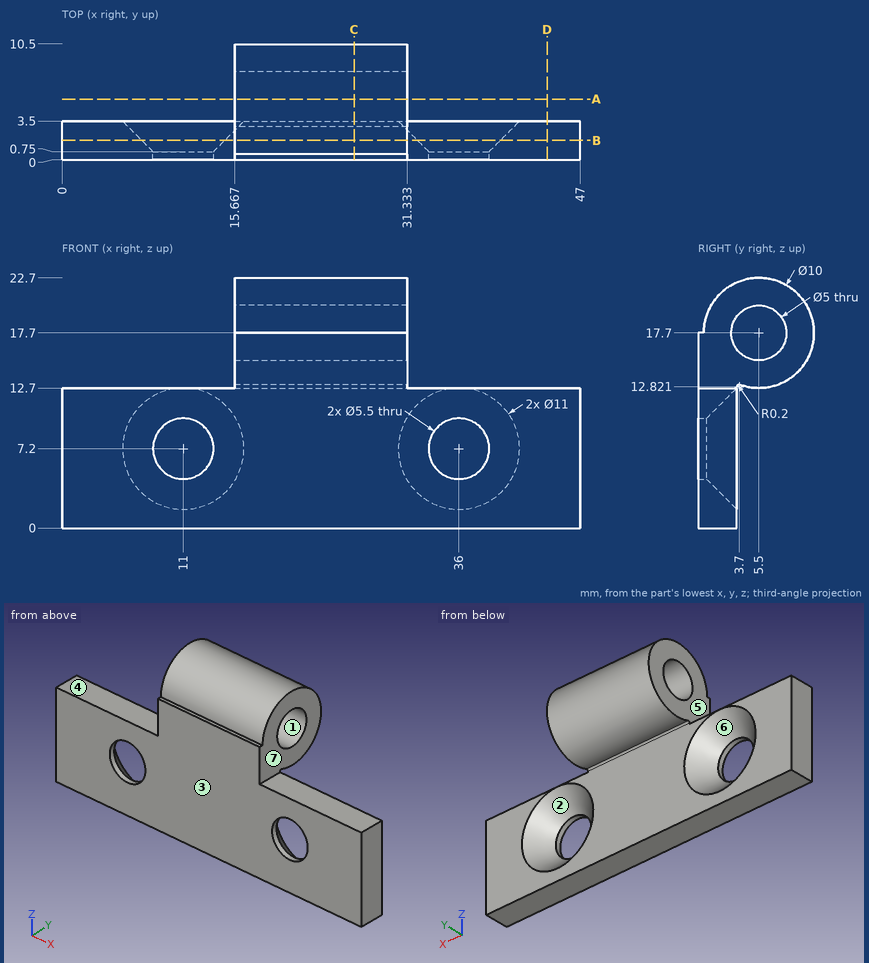
Geometry check sheet. Reference: drawing and pictorial views, mm from the part's lowest x, y, z. A direction names the side the tool comes from. Give positions to 0.01 mm unless a question says otherwise; leave off trailing zeros. Write each loop counter-clockwise with the first axis right and the second up, starting at its lowest first coordinate (ties: lowest second). Pieces come first, ordered by that corner, then holes. Notation, with made-up numbers: (89, 41) - (137, 41) arc R20 cw to (137, 71) - close; hole circle Ø3 at (71.5, 53.5). An arc over 180 degrees is marked (long way). Put each result on its own line as item: value.
Q1. Section check C-C on x = 26.5. Record the cut outline in (y, z), and give its area (3 significant figures).
Result:
outline: (0, 0) - (3.5, 0) - (3.5, 12.82) arc R0.2 cw to (3.77, 13.01) arc R5 ccw (long way) to (0.5, 17.7) - (0, 17.7) - close; hole circle Ø5 at (5.5, 17.7)
area: 111 mm2
Q2. Section check A-A on y = 5.5. Record the cut outline in (x, z).
Result:
outline: (15.67, 12.7) - (31.33, 12.7) - (31.33, 15.2) - (15.67, 15.2) - close; (15.67, 20.2) - (31.33, 20.2) - (31.33, 22.7) - (15.67, 22.7) - close
Q3. Set-up check for the marked faces 5, 6 and 7: record each of +Z, -Z, +X, -X, +Y, -Y from which the full face is reachable in a straight line by a thin tool's end or side.
Result:
face 5: +Z, -X, +Y, -Y
face 6: +Y
face 7: +Z, +X, +Y, -Y
Q4. Depth check by flat-ended pin: P1, Ø6.5, axis at x = 11, z = 7.2, coming from the +Y side; P2, Ø3, axis at x = 12.5, z = 17.5, coming from the -Y side (3 decimals); P3, Ø1.5, axis at y = 9.5, z = 14.5, coming from the -X side; P4, Ø1.8, axis at x = 7.5, y = 1.5, coming from the +Z side. Enter the tip coordinate at first touch or a pass-through.
Result:
P1: y = 1.25
P2: through
P3: x = 15.67
P4: z = 12.7
Q5. Section check B-B on y = 1.75. Record the cut outline in (x, z).
Result:
outline: (0, 0) - (47, 0) - (47, 12.7) - (31.33, 12.7) - (31.33, 21.01) - (15.67, 21.01) - (15.67, 12.7) - (0, 12.7) - close; hole circle Ø7.5 at (11, 7.2); hole circle Ø7.5 at (36, 7.2)
Q6. Scan lines: probe 1 along X at (y, z) = (0.4, 7.2); probe 2 along Z at (x, y) = (11, 0.5); probe 3 along X at (y, z) = (4.25, 21.25). Record each from-to range of solid material in increasing order. Write a range as from..to.
Result:
probe 1: 0..8.25, 13.75..33.25, 38.75..47
probe 2: 0..4.45, 9.95..12.7
probe 3: 15.67..31.33
Q7. Mould release check, pull along Y, two halves, no side actions. Record for the marked faces 1, 2, 3 and 4: released by +Y, released by -Y, zero draft, split by the parting line, or undercut.
Result:
face 1: undercut
face 2: released by +Y
face 3: released by -Y
face 4: zero draft
Q8. Section check D-D on x = 44. Record the cut outline in (y, z).
Result:
outline: (0, 0) - (3.5, 0) - (3.5, 12.7) - (0, 12.7) - close
